Source: CAD feature listing. Evaluate the final solid. Frame: model axes, mm. A direction names the side the tool comes from. Give positions to 0.01 mm unless a question says otherwise; leave off trailing zeros. Order: outer loops, then holes, each group sorted by start corner. A loop starts at its lowest first (then second) coordinate and runs counter-clockwise, first axis right, second up. Notation, with made-up numbers: M -17.75,20.25 L -9.75,20.25 A23 ccw -9.75,53.25 Z; hole C 62.5,23.25 d7. An arc over 180 degrees is marked long. Answer as a JSON object with one key per item and string values. Group by question number.
1. Set-up query: faces 1 (the conical face through (-5.62, -25.308, 14.14)), 2 (the flat face through (0, 0, 79.375)). Return all of +Z, -Z, +X, -X, +Y, -Y with unobstructed straight access to the full face (end or side cutting, diameter ignored); none if empty.
2. Section query C-C (z = 59.5). Output: boundary loops of the cut face in (x, y).
3. Pull-direction query (Z, two-part tool) for faces 3 (the cylindrical face through (-30.235, -23.183, 6.261)), 4 (the flat face through (-1, 1, 0)), 5 (the conical face through (18.53, 5.84, 39.14)); classes: +Z half, -Z half, draft (parallel to the pull), parting line (faces both ways), or undercut.
4. Material intervals for L1, parallel to Z at x = 13.5, y = -11.5; L2, parallel to Z at x = 14, y = -28; L3, parallel to Z at x = 29.5, y = -21, sorted ascending. Write a range as [from, to].
5. Pin query (flat end, axial travel): P1, Ø4, axis at x = -12, z = 65, coming from the +Y side; P2, Ø10, axis at x = 3, z = 57.5, coming from the +Y side; P3, Ø8, axis at y = -28, z = 9, coming from the -X side; P4, Ø1, axis at y = 29.5, z = 20.5, coming from the +X side. Return the tip coordinate at first contact, or that it passes through.
6. Section query B-B (z = 8). Output: boundary loops of the cut face in (x, y), plus the area to 3 significant figures.
from build123d import *

# Parameters (mm, degrees)
F0_R      = 38.1
F1_DEPTH  = 12.7
F2_R      = 25.4
F3_DEPTH  = 25.4
F3_TAPER  = -20
F4_R      = 19.05
F5_DEPTH  = 19.05
F5_TAPER  = -20
F6_R      = 12.7
F7_DEPTH  = 12.7
F7_TAPER  = -20
F8_R      = 6.35
F9_DEPTH  = 6.35
F9_TAPER  = -20
F10_R     = 3.175
F11_DEPTH = 3.175
F11_TAPER = -20


# Not quite as in the source:
# - a fillet or chamfer that OpenCascade refuses, or shapes differently, is made with other operations: its cross-section is extruded or revolved along the edge and cut away or added


with BuildPart() as f1:
    # F0 (on Top) → F1 (new body)
    with BuildSketch(Plane.XY):
        Circle(F0_R)
    extrude(amount=F1_DEPTH)

    # F2 (on face) → F3 (join)
    with BuildSketch(Plane.XY.offset(12.7)):
        Circle(F2_R)
    extrude(amount=F3_DEPTH, taper=F3_TAPER)

    # F4 (on face) → F5 (join)
    with BuildSketch(Plane.XY.offset(38.1)):
        Circle(F4_R)
    extrude(amount=F5_DEPTH, taper=F5_TAPER)

    # F6 (on face) → F7 (join)
    with BuildSketch(Plane.XY.offset(57.15)):
        Circle(F6_R)
    extrude(amount=F7_DEPTH, taper=F7_TAPER)

    # F8 (on face) → F9 (join)
    with BuildSketch(Plane.XY.offset(69.85)):
        Circle(F8_R)
    extrude(amount=F9_DEPTH, taper=F9_TAPER)

    # F10 (on face) → F11 (join)
    with BuildSketch(Plane.XY.offset(76.2)):
        Circle(F10_R)
    extrude(amount=F11_DEPTH, taper=F11_TAPER)

    # F12: chamfer of 2.54 on 5 edges, made by hand

    # F12_s1 → F12_t2 (revolve, cut)
    with BuildSketch(Plane.XZ):
        Polygon((33.7761127863, 35.7131807432), (32.1048439504, 38.1), (34.6448439504, 38.1), align=None)
    revolve(axis=Axis((0, 0, 38.1), (0, 0, -1)), mode=Mode.SUBTRACT)

    # F12_s3 → F12_t4 (revolve, cut)
    with BuildSketch(Plane.XZ):
        Polygon((25.1149017987, 54.7631807432), (23.4436329628, 57.15), (25.9836329628, 57.15), align=None)
    revolve(axis=Axis((0, 0, 57.15), (0, 0, -1)), mode=Mode.SUBTRACT)

    # F12_s5 → F12_t6 (revolve, cut)
    with BuildSketch(Plane.XZ):
        Polygon((16.4536908111, 67.4631807432), (14.7824219752, 69.85), (17.3224219752, 69.85), align=None)
    revolve(axis=Axis((0, 0, 69.85), (0, 0, -1)), mode=Mode.SUBTRACT)

    # F12_s7 → F12_t8 (revolve, cut)
    with BuildSketch(Plane.XZ):
        Polygon((7.7924798235, 73.8131807432), (6.1212109876, 76.2), (8.6612109876, 76.2), align=None)
    revolve(axis=Axis((0, 0, 76.2), (0, 0, -1)), mode=Mode.SUBTRACT)

    # F12_s9 → F12_t10 (revolve, cut)
    with BuildSketch(Plane.XZ):
        Polygon((3.4618743297, 76.9881807432), (1.7906054938, 79.375), (4.3306054938, 79.375), align=None)
    revolve(axis=Axis((0, 0, 79.375), (0, 0, -1)), mode=Mode.SUBTRACT)


solid = f1.part
Answer sheet:
{
 "1": {"face 1": "none", "face 2": "+Z, +X, -X, +Y, -Y"},
 "2": {"outline": "C 0,0 d27.11"},
 "3": {"face 3": "draft", "face 4": "-Z half", "face 5": "undercut"},
 "4": {"L1": "[0, 57.15]", "L2": "[0, 12.7], [28.92, 38.1]", "L3": "[0, 12.7]"},
 "5": {"P1": "y = 12.17", "P2": "y = 25.11", "P3": "x = -29.59", "P4": "through"},
 "6": {"outline": "C 0,0 d76.2", "area": "4,560 mm^2"}
}
